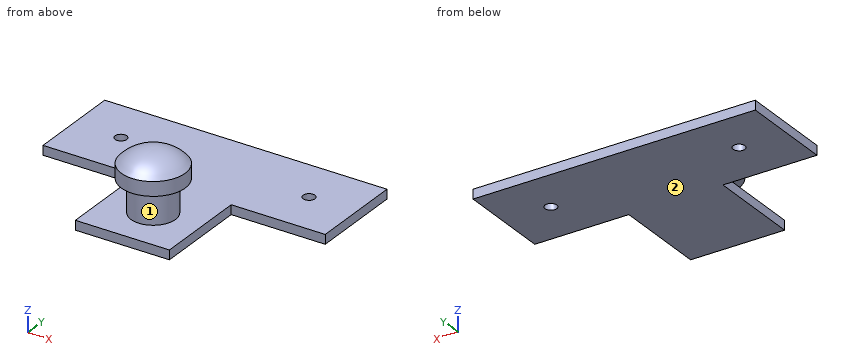
from build123d import *

# Parameters (mm, degrees)
BOSS_EXTRUDE1_DEPTH = 2.54
SKETCH2_R           = 6
BOSS_EXTRUDE2_DEPTH = 8.89
CUT_EXTRUDE1_REACH  = 20.872
SKETCH5_R           = 1.5875


with BuildPart() as part:
    # Sketch1 → Boss-Extrude1 (new body)
    with BuildSketch(Plane.XY):
        Polygon((12.7, 0), (38.1, 0), (38.1, 25.4), (-38.1, 25.4), (-38.1, 0), (-12.7, 0), (-12.7, -25.4), (12.7, -25.4), align=None)
    extrude(amount=BOSS_EXTRUDE1_DEPTH)

    # Sketch2 → Boss-Extrude2 (add)
    with BuildSketch(Plane.XY.offset(2.54)):
        with Locations((0, -12.7)):
            Circle(SKETCH2_R)
    extrude(amount=BOSS_EXTRUDE2_DEPTH)

    # Sketch4 → Revolve1 (revolve)
    with BuildSketch(Plane(origin=(0, 0, 0), x_dir=(0, 0, -1), z_dir=(1, 0, 0))):
        with BuildLine():
            Line((-11.43, -12.7), (-18.854523239, -12.7))
            ThreePointArc((-18.854523239, -12.7), (-18.044308382, -17.435305314), (-15.24, -21.336))
            Line((-15.24, -21.336), (-11.43, -21.336))
            Line((-11.43, -21.336), (-11.43, -12.7))
        make_face()
    revolve(axis=Axis((0, -12.7, 11.43), (0, 0, 1)))

    # Sketch5 → Cut-Extrude1 (cut, up to next)
    with BuildSketch(Plane(origin=(0, 0, 0), x_dir=(-1, 0, 0), z_dir=(0, 0, -1)), mode=Mode.PRIVATE) as cut_extrude1_sk1:
        with Locations((25.4, 12.7)):
            Circle(SKETCH5_R)
    cut_extrude1_tool1 = extrude(cut_extrude1_sk1.sketch, amount=-CUT_EXTRUDE1_REACH, mode=Mode.PRIVATE) & part.part
    add(cut_extrude1_tool1.solids().sort_by_distance((-25.4, 12.7, 0))[0], mode=Mode.SUBTRACT)
    # Sketch5 → Cut-Extrude1 (cut, up to next)
    with BuildSketch(Plane(origin=(0, 0, 0), x_dir=(-1, 0, 0), z_dir=(0, 0, -1)), mode=Mode.PRIVATE) as cut_extrude1_sk2:
        with Locations((-25.4, 12.7)):
            Circle(SKETCH5_R)
    cut_extrude1_tool2 = extrude(cut_extrude1_sk2.sketch, amount=-CUT_EXTRUDE1_REACH, mode=Mode.PRIVATE) & part.part
    add(cut_extrude1_tool2.solids().sort_by_distance((25.4, 12.7, 0))[0], mode=Mode.SUBTRACT)


solid = part.part
Input: part model. Units: mm. Frame: model coordinates. Face numbers are marked on the shaded views. Round coordinates to 2 decimals unless told otherwise and drop trailing zeros. Write each loop counter-clockwise with the first axis right and the second up, starting at its lowest first coordinate (ties: lowest second). Pieces come first, ordered by that corner, then holes.
1) Ray query, L1, parallel to Y at x = -25.4, z = 0.65; L2, parallel to Z at x = 31.5, y = 11; L3, parallel to Y at x = -4.5, z = 3.75. Return the intervals inside material, ascending.
2) Contact query for flat-ended pins moving along their axis: P1, Ø3, axis at x = 26.5, z = 1.5, coming from the -Y side; P2, Ø0.8, axis at y = -12.5, z = 2, coming from the +X side; P3, Ø8, axis at y = -13, z = 3.5, coming from the -X side. Output: stop coordinate, or through.
3) Draft query along Z for the marked faces 1 and 2. Return one class per face: pulls with the +Z half, pulls with the -Z half, needs draft (parallel to the pull), parting line crosses it, or undercut.
4) Cut plane B-B (y = 12.7). Return the cut outline in (x, z), then the cut area to 3 significant figures.
5) Cut plane A-A (x = -25.4). Return the cut outline in (y, z).
6) Cut plane D-D (y = 6). Return the cut outline in (x, z), then the cut area to 3 significant figures.
7) Cut plane C-C (z = 7.5). Return the cut outline in (x, y), then the cut area to 3 significant figures.
Geometry says:
1. L1: y = 0 to 11.11, 14.29 to 25.4
1. L2: z = 0 to 2.54
1. L3: y = -16.67 to -8.73
2. P1: stops at y = 0
2. P2: stops at x = 12.7
2. P3: stops at x = -12.7
3. face 1: undercut
3. face 2: pulls with the -Z half
4. outline: (-38.1, 0) - (-26.99, 0) - (-26.99, 2.54) - (-38.1, 2.54) - close; (-23.81, 0) - (23.81, 0) - (23.81, 2.54) - (-23.81, 2.54) - close; (26.99, 0) - (38.1, 0) - (38.1, 2.54) - (26.99, 2.54) - close
4. area: 177 mm2
5. outline: (0, 0) - (11.11, 0) - (11.11, 2.54) - (0, 2.54) - close; (14.29, 0) - (25.4, 0) - (25.4, 2.54) - (14.29, 2.54) - close
6. outline: (-38.1, 0) - (38.1, 0) - (38.1, 2.54) - (-38.1, 2.54) - close
6. area: 194 mm2
7. outline: circle Ø12 at (0, -12.7)
7. area: 113 mm2
